Could you check a few things on this drawing? It's one solid part, dimensions in mm from its lowest x, y, z. Give positions to 0.01 mm unless a question says otherwise; leave off trailing zeros. Loops run counter-clockwise (first coordinate to the right, second up) from the corner with the lowest first, then second, coordinate; pieces in that order, holes last. Notation, with made-up numbers: (22.25, 88.5) - (31.25, 88.5) arc R35 cw to (31.25, 124.5) - close; hole circle Ø3 at (34.25, -15). An arc over 180 degrees is marked (long way). Use a Markdown table: item, result.
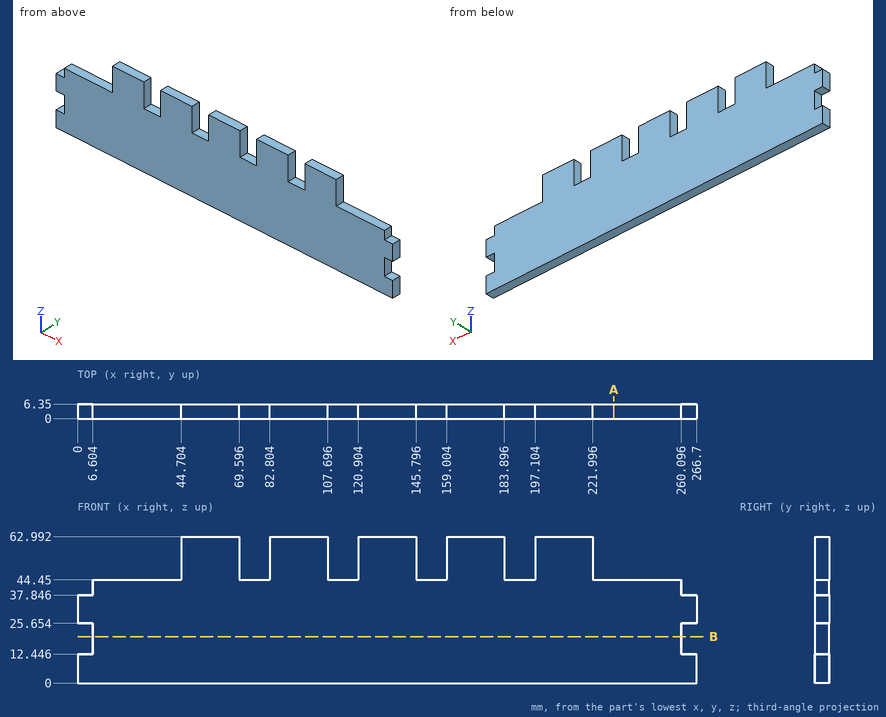
(1) Suppose I cut it at B-B on z = 20. Write out the boundary of the cut face in (x, y).
A:
| item | result |
|---|---|
| outline | (6.6, 0) - (260.1, 0) - (260.1, 6.35) - (6.6, 6.35) - close |
(2) If I drill on line 1 (X direction, y = 6.25, z = 50.5); line 2 (X direction, y = 4.25, z = 20); line 3 (Z direction, x = 227.5, y = 1), over which ranges is the centre line in solid material (lowest first)?
A:
| item | result |
|---|---|
| line 1 | 44.7 to 69.6, 82.8 to 107.7, 120.9 to 145.8, 159 to 183.9, 197.1 to 222 |
| line 2 | 6.6 to 260.1 |
| line 3 | 0 to 44.45 |
(3) Will these pins go through, and if not, where does the flat tip stop? pin 1 (3 mm diameter, centred on y = 3.5, z = 58, fed in from -X); pin 2 (3 mm diameter, centred on y = 2.5, z = 51.5, fed in from +X); pin 3 (1.9 mm diameter, centred on x = 20, y = 2.5, fed in from +Z).
A:
| item | result |
|---|---|
| pin 1 | x = 44.7 |
| pin 2 | x = 222 |
| pin 3 | z = 44.45 |
(4) Suppose I cut it at A-A on x = 231. Write out the boundary of the cut face in (y, z), plus the area to 3 significant figures.
A:
| item | result |
|---|---|
| outline | (0, 0) - (6.35, 0) - (6.35, 44.45) - (0, 44.45) - close |
| area | 282 mm2 |
